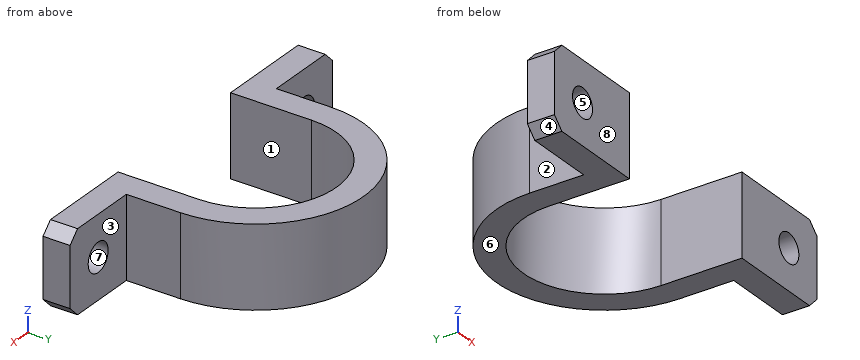
from build123d import *

# Parameters (mm, degrees)
PAD_DEPTH    = 19.05
SKETCH001_R  = 3.3782
HOLE_DEPTH   = 24.9936
CHAMFER_SIZE = 2.54


with BuildPart() as part:
    # Sketch → Pad (new body)
    with BuildSketch(Plane.XY):
        with BuildLine():
            ThreePointArc((19.05, 0), (0, 19.05), (-19.05, 0))
            Line((-19.05, 0), (-19.05, -19.05))
            Line((-19.05, -19.05), (-25.4, -19.05))
            Line((-44.45, -19.05), (-25.4, -19.05))
            Line((-44.45, -12.7), (-44.45, -19.05))
            Line((-25.4, -12.7), (-44.45, -12.7))
            Line((-25.4, -12.7), (-25.4, 0))
            ThreePointArc((25.4, 0), (0, 25.4), (-25.4, 0))
            Line((25.4, 0), (25.4, -12.7))
            Line((25.4, -12.7), (44.45, -12.7))
            Line((44.45, -12.7), (44.45, -19.05))
            Line((44.45, -19.05), (25.4, -19.05))
            Line((19.05, -19.05), (25.4, -19.05))
            Line((19.05, 0), (19.05, -19.05))
        make_face()
    extrude(amount=PAD_DEPTH)

    # Sketch001 → Hole (cut)
    with BuildSketch(Plane.XZ):
        with Locations((34.925, 9.525)):
            Circle(SKETCH001_R)
        with Locations((-34.925, 9.525)):
            Circle(SKETCH001_R)
    extrude(amount=HOLE_DEPTH, mode=Mode.SUBTRACT)

    # Chamfer
    chamfer_edges = [part.edges().sort_by_distance(p)[0] for p in [
        (-44.45, -15.875, 19.05),
        (-44.45, -15.875, 0),
        (44.45, -15.875, 0),
        (44.45, -15.875, 19.05),
    ]]
    chamfer(chamfer_edges, length=CHAMFER_SIZE)


solid = part.part
Part model, mm, in its own coordinate system. Face numbers are marked on the shaded views. A direction names the side the tool comes from. Round coordinates to 2 decimals unless told otherwise and drop trailing zeros. Write each loop counter-clockwise with the first axis right and the second up, starting at its lowest first coordinate (ties: lowest second). Pieces come first, ordered by that corner, then holes. Notation, with made-up numbers: M 42.25,14.25 L 76.25,14.25 A18 ccw 76.25,43.25 Z; hole C 83.5,78.5 d2. An arc over 180 degrees is marked long. Return JSON: item names as keys, results as strings. Group by question number.
(1) Which spindle directions (+Z, -Z, +X, -X, +Y, -Y) get a long thin tool onto all of the face, cutting with end or side? Do the marked faces 1, 2, 3 and 4. Say none if no direction does.
(2) Saw through at B-B on x = 35. Write the cut outline in (y, z), then the cut area to 3 significant figures.
(3) Saw through at D-D on z = 15.25. Write the cut outline in (x, y).
(4) Saw through at A-A on y = -9.5. Write the cut outline in (x, z), then the cut area to 3 significant figures.
(5) Saw through at C-C on z = 7.5. Write the cut outline in (x, y), then the cut area to 3 significant figures.
(6) Drill centre lines: probe 1 along X at (y, z) = (-13, 10.5); probe 2 along X at (y, z) = (-17, 4.75); probe 3 along X at (y, z) = (-15, 10). Where is each one in solid material? Low to high.
(7) Pin check, flat tips, straight feed: pin 1 Ø5.5 at (x, z) = (38.5, 7) entering from +Y; pin 2 Ø1.5 at (y, z) = (7.5, 10.5) entering from +X; pin 3 Ø4 at (y, z) = (-8.5, 11.5) entering from +X; pin 4 Ø5.5 at (x, z) = (-34.925, 9.525) entering from -Y. Stop position of each tip, or through.
(8) Two-plate mould, pull along Z, no slides. Class the marked faces 5, 6, 7 and 8: +Z half, -Z half, draft (parallel to the pull), parting line (faces both ways), or undercut.
Returned:
{
 "1": {"face 1": "+Z, -Z, -Y", "face 2": "+Z, -Z, -X, +Y", "face 3": "+Z, -Z, +X, +Y", "face 4": "-Z, -X, +Y, -Y"},
 "2": {"outline": "M -19.05,0 L -12.7,0 L -12.7,6.15 L -19.05,6.15 Z; M -19.05,12.9 L -12.7,12.9 L -12.7,19.05 L -19.05,19.05 Z", "area": "78.1 mm²"},
 "3": {"outline": "M -44.45,-19.05 L -19.05,-19.05 L -19.05,0 A19.05 cw 19.05,0 L 19.05,-19.05 L 44.45,-19.05 L 44.45,-12.7 L 25.4,-12.7 L 25.4,0 A25.4 ccw -25.4,0 L -25.4,-12.7 L -44.45,-12.7 Z"},
 "4": {"outline": "M -25.4,0 L -19.05,0 L -19.05,19.05 L -25.4,19.05 Z; M 19.05,0 L 25.4,0 L 25.4,19.05 L 19.05,19.05 Z", "area": "242 mm²"},
 "5": {"outline": "M -44.45,-19.05 L -37.63,-19.05 L -37.63,-12.7 L -44.45,-12.7 Z; M -32.22,-19.05 L -19.05,-19.05 L -19.05,0 A19.05 cw 19.05,0 L 19.05,-19.05 L 32.22,-19.05 L 32.22,-12.7 L 25.4,-12.7 L 25.4,0 A25.4 ccw -25.4,0 L -25.4,-12.7 L -32.22,-12.7 Z; M 37.63,-19.05 L 44.45,-19.05 L 44.45,-12.7 L 37.63,-12.7 Z", "area": "859 mm²"},
 "6": {"probe 1": "-44.45 to -38.16, -31.69 to -19.05, 19.05 to 31.69, 38.16 to 44.45", "probe 2": "-44.45 to -19.05, 19.05 to 44.45", "probe 3": "-44.45 to -38.27, -31.58 to -19.05, 19.05 to 31.58, 38.27 to 44.45"},
 "7": {"pin 1": "y = -12.7", "pin 2": "x = 24.49", "pin 3": "x = 25.4", "pin 4": "through"},
 "8": {"face 5": "undercut", "face 6": "-Z half", "face 7": "undercut", "face 8": "draft"}
}
